```python
from build123d import *

# Parameters (mm, degrees)
EXTRUDE_1_DEPTH              = 3
FILLET_1_R                   = 2
HOLE_WIZARD_M4_1_D           = 4.5
HOLE_WIZARD_M4_1_DEPTH       = 24.5
HOLE_WIZARD_M4_1_CSINK_D     = 9.18
HOLE_WIZARD_M4_1_CSINK_ANGLE = 90
HOLE_WIZARD_M4_1_TIP         = 1.351936393
HOLE_WIZARD_M3_1_D           = 3.4
HOLE_WIZARD_M3_1_DEPTH       = 24.5
HOLE_WIZARD_M3_1_CSINK_D     = 6.94
HOLE_WIZARD_M3_1_CSINK_ANGLE = 90
HOLE_WIZARD_M3_1_TIP         = 1.021463052
EXTRUDE_START                = -3
EXTRUDE_2_DEPTH              = 3
FILLET_2_R                   = 3


with BuildPart() as part:
    # 草图1 → 凸台-拉伸1 (new body)
    with BuildSketch(Plane.XY):
        Polygon((0, 0), (-15, 0), (-15, 26.213203436), (20, 61.213203436), (20, 81.213203436), (35, 81.213203436), (35, 55), (0, 20), align=None)
    extrude(amount=EXTRUDE_1_DEPTH)

    # 圆角1
    fillet_1_edges = [part.edges().sort_by_distance(p)[0] for p in [
        (0, 0, 1.5),
        (-15, 0, 1.5),
        (-15, 26.213203436, 1.5),
        (20, 61.213203436, 1.5),
        (20, 81.213203436, 1.5),
        (35, 81.213203436, 1.5),
        (35, 55, 1.5),
        (0, 20, 1.5),
    ]]
    fillet(fillet_1_edges, radius=FILLET_1_R)

    # M4 六角凹锥坑头螺钉的锥形沉头孔1
    with Locations(Plane(origin=(27.5, 76.213203436, 0), x_dir=(-1, 0, 0), z_dir=(0, 0, -1))):
        with Locations((0, 0), (0, -10), (35, -61.213203436), (35, -71.213203436)):
            CounterSinkHole(HOLE_WIZARD_M4_1_D / 2, HOLE_WIZARD_M4_1_CSINK_D / 2, depth=HOLE_WIZARD_M4_1_DEPTH, counter_sink_angle=HOLE_WIZARD_M4_1_CSINK_ANGLE)
            with Locations((0, 0, -(HOLE_WIZARD_M4_1_DEPTH + HOLE_WIZARD_M4_1_TIP / 2))):  # 118° drill point
                Cone(0, HOLE_WIZARD_M4_1_D / 2, HOLE_WIZARD_M4_1_TIP, mode=Mode.SUBTRACT)

    # M3 六角凹锥坑头螺钉的锥形沉头孔1
    with Locations(Plane(origin=(15.656854249, 46.263455967, 0), x_dir=(-1, 0, 0), z_dir=(0, 0, -1))):
        with Locations((0, 0), (11.313708498, -11.313708499)):
            CounterSinkHole(HOLE_WIZARD_M3_1_D / 2, HOLE_WIZARD_M3_1_CSINK_D / 2, depth=HOLE_WIZARD_M3_1_DEPTH, counter_sink_angle=HOLE_WIZARD_M3_1_CSINK_ANGLE)
            with Locations((0, 0, -(HOLE_WIZARD_M3_1_DEPTH + HOLE_WIZARD_M3_1_TIP / 2))):  # 118° drill point
                Cone(0, HOLE_WIZARD_M3_1_D / 2, HOLE_WIZARD_M3_1_TIP, mode=Mode.SUBTRACT)

    # 草图5 → 凸台-拉伸2 (add)
    with BuildSketch(Plane(origin=(0, 0, 0), x_dir=(-1, 0, 0), z_dir=(0, 0, -1)).offset(EXTRUDE_START)):
        with BuildLine():
            Line((-33, 81.213203436), (-50, 81.213203436))
            Line((-50, 81.213203436), (-50, 70))
            Line((-50, 70), (-34.414213562, 54.414213562))
            ThreePointArc((-34.414213562, 54.414213562), (-34.847759065, 55.06306026), (-35, 55.828427125))
            Line((-35, 55.828427125), (-35, 79.213203436))
            ThreePointArc((-35, 79.213203436), (-34.414213562, 80.627416998), (-33, 81.213203436))
        make_face()
    extrude(amount=EXTRUDE_2_DEPTH)

    # 圆角2
    fillet_2_edges = [part.edges().sort_by_distance(p)[0] for p in [
        (50, 70, 1.5),
        (50, 81.213203436, 1.5),
    ]]
    fillet(fillet_2_edges, radius=FILLET_2_R)


solid = part.part
```
The listing builds one solid part. Answer for the finished solid, in the listing's coordinates (mm). A direction names the side the tool comes from. Round coordinates to 2 decimals unless told otherwise and drop trailing zeros. Loops run counter-clockwise (first coordinate to the right, second up) from the corner with the lowest first, then second, coordinate; pieces in that order, holes last.
1) For faces 1 (the face through (0, 11, 1)), 2 (the face through (-7.988, 12.804, 2.675)), 3 (the face through (20, 71, 1)), determine the directions among +Z, -Z, +X, -X, +Y, -Y from which every point of the face is accessible in a straight line to the end or side of a thin tool.
Outcome:
face 1: +Z, -Z, +X, -Y
face 2: +Z, -Z
face 3: +Z, -Z, -X, +Y
2) A cutting plane is placed at D-D on x = 33.5. Determine the outline of the cut face in (y, z).
Outcome:
outline: (53.5, 0) - (81.21, 0) - (81.21, 3) - (53.5, 3) - close
3) A cutting plane is placed at B-B on x = -7.5. Determine the outline of the cut face in (y, z), plus the area to 3 significant figures.
Outcome:
outline: (0, 0) - (0.41, 0) - (2.75, 2.34) - (2.75, 3) - (0, 3) - close; (7.25, 2.34) - (9.59, 0) - (10.41, 0) - (12.75, 2.34) - (12.75, 3) - (7.25, 3) - close; (17.25, 2.34) - (19.59, 0) - (33.71, 0) - (33.71, 3) - (17.25, 3) - close
area: 63.2 mm2
4) A cutting plane is placed at C-C on z = 0.9. Determine the outline of the cut face in (x, y).
Outcome:
outline: (-15, 2) arc R2 ccw to (-13, 0) - (-2, 0) arc R2 ccw to (0, 2) - (0, 19.17) arc R2 cw to (0.59, 20.59) - (49.12, 69.12) arc R3 ccw to (50, 71.24) - (50, 78.21) arc R3 ccw to (47, 81.21) - (22, 81.21) arc R2 ccw to (20, 79.21) - (20, 62.04) arc R2 cw to (19.41, 60.63) - (-14.41, 26.8) arc R2 ccw to (-15, 25.38) - close; hole circle Ø7.38 at (-7.5, 5); hole circle Ø7.38 at (-7.5, 15); hole circle Ø5.14 at (4.34, 34.95); hole circle Ø5.14 at (15.66, 46.26); hole circle Ø7.38 at (27.5, 66.21); hole circle Ø7.38 at (27.5, 76.21)
5) For a pull along X with two mould halves and no side action, classify faces 4 (the face through (25, 45, 2)), 5 (the face through (18, 44, 3)), 6 (the face through (2.263, 43.476, 1.479)), 7 (the face through (13.96, 46.34, 2.39)) as released by +X, released by -X, zero draft, split by the parting line, or undercut.
Outcome:
face 4: released by +X
face 5: zero draft
face 6: released by -X
face 7: undercut
6) A cutting plane is placed at A-A on y = 15. Determine the outline of the cut face in (x, z).
Outcome:
outline: (-15, 0) - (-12.09, 0) - (-9.75, 2.34) - (-9.75, 3) - (-15, 3) - close; (-5.25, 2.34) - (-2.91, 0) - (0, 0) - (0, 3) - (-5.25, 3) - close
7) Given P1, Ø5.5, axis at x = 15.66, y = 46.26, coming from the -Z side; P2, Ø4, axis at x = 27.5, y = 76.21, coming from the +Z side; P3, Ø1.5, axis at x = 13, z = 2, coming from the +Y side; P4, Ø1.5, axis at y = 14.5, z = 2, coming from the +X side, each flat-ended and moving along its own axis, determine where each tip first touches the part or whether it passes through.
Outcome:
P1: stops at z = 0.72
P2: passes through
P3: stops at y = 54.96
P4: stops at x = 0
8) Consider line 1 (Y direction, x = 27.5, z = 2.5); line 2 (X direction, y = 15, z = 2.7); line 3 (Y direction, x = 5, z = 0.8). Determine where each line is inside the solid, lowest interval first.
Outcome:
line 1: y = 47.5 to 63.96, 68.46 to 73.96, 78.46 to 81.21
line 2: x = -15 to -9.75, -5.25 to 0
line 3: y = 25 to 32.36, 37.54 to 46.21
